from build123d import *

# Parameters (mm, degrees)
SKETCH1_W           = 25.4
SKETCH1_H           = 25.4
SKETCH1_W_2         = 19.05
SKETCH1_H_2         = 19.05
BOSS_EXTRUDE1_DEPTH = 127
SKETCH3_R           = 2.0193
CUT_EXTRUDE1_DEPTH  = 26.4
LPATTERN1_COUNT     = 20
LPATTERN1_PITCH     = 12.7
SKETCH4_R           = 2.0193
CUT_EXTRUDE2_DEPTH  = 26.4
LPATTERN2_COUNT     = 20
LPATTERN2_PITCH     = 12.7
SKETCH8_R           = 14.2875
CUT_EXTRUDE6_DEPTH  = 3.175


with BuildPart() as part:
    # Sketch1 → Boss-Extrude1 (new body, symmetric)
    with BuildSketch(Plane.XY):
        Rectangle(SKETCH1_W, SKETCH1_H)
        Rectangle(SKETCH1_W_2, SKETCH1_H_2, mode=Mode.SUBTRACT)
    extrude(amount=BOSS_EXTRUDE1_DEPTH, both=True)

    # Sketch3 → Cut-Extrude1 (cut, through all)
    with BuildSketch(Plane(origin=(0, 12.7, 0), x_dir=(1, 0, 0), z_dir=(0, 1, 0))):
        with Locations((0, -120.65)):
            Circle(SKETCH3_R)
    cut_extrude1 = extrude(amount=-CUT_EXTRUDE1_DEPTH, mode=Mode.SUBTRACT)

    # LPattern1: Cut-Extrude1 ×20
    with Locations(*[(0, 0, -i * LPATTERN1_PITCH) for i in range(1, LPATTERN1_COUNT)]):
        add(cut_extrude1, mode=Mode.SUBTRACT)

    # Sketch4 → Cut-Extrude2 (cut, through all)
    with BuildSketch(Plane.ZY.offset(12.7)):
        with Locations((120.65, 0)):
            Circle(SKETCH4_R)
    cut_extrude2 = extrude(amount=-CUT_EXTRUDE2_DEPTH, mode=Mode.SUBTRACT)

    # LPattern2: Cut-Extrude2 ×20
    with Locations(*[(0, 0, -i * LPATTERN2_PITCH) for i in range(1, LPATTERN2_COUNT)]):
        add(cut_extrude2, mode=Mode.SUBTRACT)

    # Sketch8 → Cut-Extrude6 (cut)
    with BuildSketch(Plane(origin=(0, 12.7, 0), x_dir=(1, 0, 0), z_dir=(0, 1, 0))):
        with Locations((0, 25.4)):
            Circle(SKETCH8_R)
    cut_extrude6 = extrude(amount=-CUT_EXTRUDE6_DEPTH, mode=Mode.SUBTRACT)

    # Mirror4: Cut-Extrude6 across plane
    add(cut_extrude6.mirror(Plane.ZX), mode=Mode.SUBTRACT)


solid = part.part
Verification items for the finished model (mm, model axes). A direction names the side the tool comes from. Coordinates: 2 decimals unless noted, no trailing zeros. Loops run counter-clockwise (first coordinate to the right, second up) from the corner with the lowest first, then second, coordinate; pieces in that order, holes last. Notation, with made-up numbers: M -12.5,29 L 29.5,29 A28 ccw 29.5,67 Z; hole C 52.5,-30.75 d10. An arc over 180 degrees is marked long. One line per item, written item: value.
1. Section check C-C on x = 4.5. Record the cut outline in (y, z) (3 decimals), plus the area to 3 significant figures.
Answers follow:
outline: M -12.7,-127 L -9.525,-127 L -9.525,-38.96 L -12.7,-38.96 Z; M -12.7,-11.84 L -9.525,-11.84 L -9.525,127 L -12.7,127 Z; M 9.525,-127 L 12.7,-127 L 12.7,-38.96 L 9.525,-38.96 Z; M 9.525,-11.84 L 12.7,-11.84 L 12.7,127 L 9.525,127 Z
area: 1,440 mm^2
2. Material ranges on line 1 along Y through (x, z) = (-2.75, 90.5) (3 decimals); line 2 along Y through (x, z) = (-11, 57.5), recorded low to high. Write a range as from..to.
Answers follow:
line 1: -12.7..-9.525, 9.525..12.7
line 2: -12.7..-1.99, 1.99..12.7
3. Set-up check for faces 1 (the cylindrical face through (-0.44, -11.09, 122.62)), 2 (the cylindrical face through (0.219, 11.135, -39.686)), 3 (the flat face through (-2.3, 9.525, 57.1)): record each of +Z, -Z, +X, -X, +Y, -Y from which the full face is reachable in a straight line by a thin tool's end or side.
Answers follow:
face 1: +Y, -Y
face 2: +Y
face 3: +Z, -Z
4. Section check B-B on y = -6.25. Record the cut outline in (x, z) (3 decimals), plus the area to 3 significant figures.
Answers follow:
outline: M -12.7,-127 L -9.525,-127 L -9.525,127 L -12.7,127 Z; M 9.525,-127 L 12.7,-127 L 12.7,127 L 9.525,127 Z
area: 1,610 mm^2
5. Section check A-A on z = -78. Record the cut outline in (x, y) (3 decimals).
Answers follow:
outline: M -12.7,-12.7 L 12.7,-12.7 L 12.7,12.7 L -12.7,12.7 Z; hole M -9.525,-9.525 L 9.525,-9.525 L 9.525,9.525 L -9.525,9.525 Z
6. Mould release check, pull along X, two halves, no side actions. Record for faces 4 (the flat face through (-3, -12.7, 55)), 5 (the cylindrical face through (-0.44, 11.13, -42.48)): pulls with the +X half, pulls with the -X half, needs draft (parallel to the pull), parting line crosses it, or undercut.
Answers follow:
face 4: needs draft
face 5: undercut
